Model file for the job. Use its own axes, mm. Face numbers are marked on the shaded views. A direction names the side the tool comes from. Give positions to 0.01 mm unless a question says otherwise; leave off trailing zeros. Loops run counter-clockwise (first coordinate to the right, second up) from the corner with the lowest first, then second, coordinate; pieces in that order, holes last. Notation, with made-up numbers: (31, 70) - (45, 70) arc R19 cw to (45, 84) - close; hole circle Ø8 at (36, 58.5). An arc over 180 degrees is marked (long way). Answer as CSV lines item,"result". Start each with the question number.
Item 1: Drill centre lines: L1, parallel to X at y = -7, z = 13; L2, parallel to Y at x = -32.5, z = 9.75; L3, parallel to Y at x = -37, z = 7.25. Where is each one in solid material? Low to high. Write a range as from..to.
Item 2: Saw through at D-D on z = 2.25. Give the cut face in (x, y).
Item 3: Saw through at A-A on y = 14. Give the cut face in (x, z), plus the area to 3 significant figures.
Item 4: Saw through at B-B on x = -18.5. Give the cut face in (y, z).
Item 5: Tool access for the marked faces 1, 2 and 3: list every direction of +Z, -Z, +X, -X, +Y, -Y with a clear straight run to the whole face (end or side of a thin tool).
Item 6: Pull direction Y, two halves, no side cores. Call the marked faces 4, 5 and 6: pulls with the +Y half, pulls with the -Y half, needs draft (parallel to the pull), parting line crosses it, or undercut.
Item 7: Pin check, flat tips, straight feed: pin 1 (8 mm diameter, centred on x = -17, y = 8, fed in from -Z); pin 2 (3 mm diameter, centred on x = -26.5, z = 17.5, fed in from +Y); pin 3 (10 mm diameter, centred on x = -16, z = 9, fed in from +Y). Stop position of each tip, or through.
Item 8: Saw through at C-C on z = 10. Give the cut face in (x, y), plus the area to 3 significant figures.
from build123d import *

# Parameters (mm, degrees)
BOSS_EXTRUDE1_DEPTH = 20
SKETCH2_R           = 5
BOSS_EXTRUDE2_DEPTH = 72.120579


with BuildPart() as part:
    # Sketch1 → Boss-Extrude1 (new body)
    with BuildSketch(Plane.XY):
        Polygon((-51.698191127, 23.057124059), (-51.698191127, -36.942875941), (20.422387717, -36.942875941), (20.422387717, 23.057124059), (10.422387717, 23.057124059), (10.422387717, -33.942875941), (-41.698191127, -33.942875941), (-41.698191127, 23.057124059), align=None)
    extrude(amount=BOSS_EXTRUDE1_DEPTH)

    # Sketch2 → Boss-Extrude2 (add)
    with BuildSketch(Plane(origin=(20.422387717, 0, 0), x_dir=(0, 0, -1), z_dir=(1, 0, 0))):
        with Locations(Location((-10, 8.057124059, 0), (0, 0, 90))):
            Circle(SKETCH2_R)
    extrude(amount=-BOSS_EXTRUDE2_DEPTH)


solid = part.part
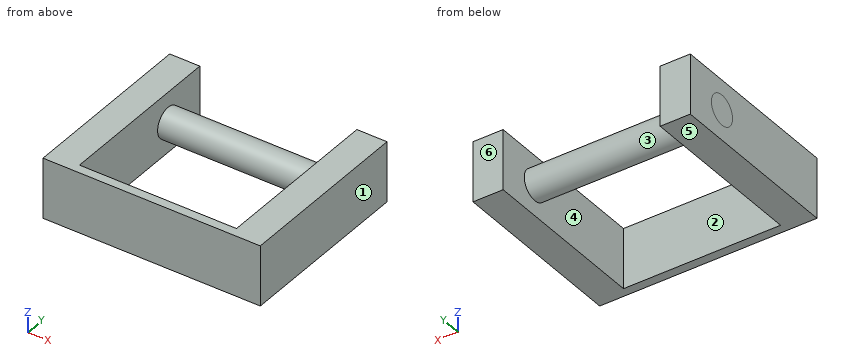
Responses:
1,L1,"-51.7..-41.7, 10.42..20.42"
1,L2,"-36.94..-33.94, 3.06..13.05"
1,L3,"-36.94..-33.94, 3.88..12.23"
2,outline,"(-51.7, -36.94) - (20.42, -36.94) - (20.42, 23.06) - (10.42, 23.06) - (10.42, -33.94) - (-41.7, -33.94) - (-41.7, 23.06) - (-51.7, 23.06) - close"
3,outline,"(-51.7, 0) - (-41.7, 0) - (-41.7, 20) - (-51.7, 20) - close; (10.42, 0) - (20.42, 0) - (20.42, 20) - (10.42, 20) - close"
3,area,"400 mm2"
4,outline,"(-36.94, 0) - (-33.94, 0) - (-33.94, 20) - (-36.94, 20) - close; circle Ø10 at (8.06, 10)"
5,face 1,"+Z, -Z, +X, +Y, -Y"
5,face 2,"+Z, -Z"
5,face 3,"none"
6,face 4,"undercut"
6,face 5,"needs draft"
6,face 6,"pulls with the +Y half"
7,pin 1,"z = 5"
7,pin 2,"y = -33.94"
7,pin 3,"y = 13.06"
8,outline,"(-51.7, -36.94) - (20.42, -36.94) - (20.42, 23.06) - (10.42, 23.06) - (10.42, 13.06) - (-41.7, 13.06) - (-41.7, 23.06) - (-51.7, 23.06) - close; hole (-41.7, -33.94) - (10.42, -33.94) - (10.42, 3.06) - (-41.7, 3.06) - close"
8,area,"1,880 mm2"
